The listing builds one solid part. Answer for the finished solid, in the listing's coordinates (mm). A direction names the side the tool comes from. Round coordinates to 2 decimals unless told otherwise and drop trailing zeros. Order: outer loops, then holes, each group sorted by start corner. A loop starts at its lowest first (then second) coordinate and runs counter-clockwise, first axis right, second up. Notation, with made-up numbers: (-35, -25) - (-13, -25) arc R22 ccw to (-13, 8) - close; hole circle Ø7 at (-36.75, 53). An arc over 180 degrees is marked (long way). Use CSV: the item, a comma, the result in double quotes. Start each with the question number.
Item 1: Determine the mould class of faces 1 (the cylindrical face through (847.575, 49.3, -6.509)), 2 (the flat face through (739, 49, 85)), 3 (the cylindrical face through (-39.05, 49.3, -8.67)), 4 (the cylindrical face through (882.98, 49.3, -1.87)) for opening direction X: +X half, -X half, draft (parallel to the pull), parting line (faces both ways), or undercut.
Item 2: Straight lines are drawn through the part: line 1 along X through (y, z) = (62, 0); line 2 along X through (y, z) = (68, -22); line 3 along Z through (x, y) = (282, 81.5). For each, find the intervals that lie inside material, in ascending order. Write a range as [from, to].
Item 3: Find section A-A, the plane z = 0. Give the vertices of the cut face in (x, y).
Item 4: Find section B-B, the plane y = 46. Give the vertices of the cut face in (x, z).
Item 5: Flat-ended cylindrical pins translate along their axes: P1, Ø8, axis at y = 30, z = 39, coming from the +X side; P2, Ø3, axis at x = 453.5, y = 14.5, coming from the -Z side; P3, Ø1.5, axis at y = 56.5, z = -33.5, coming from the -X side. Find the tip coordinate at first contact, or state that the pin passes through.
Item 6: Find section C-C, the plane x = 304. Give the vertices of the cut face in (y, z), plus the area to 3 significant figures.
Item 7: For faces 5 (the flat face through (403, 49, 65)), 6 (the cylindrical face through (669.13, 49.3, -70.484)), 7 (the flat face through (406, 100, 1)), determine the directions among +Z, -Z, +X, -X, +Y, -Y from which every point of the face is accessible in a straight line to the end or side of a thin tool.
```python
from build123d import *

# Parameters (mm, degrees)
SKETCH1_R           = 50
SKETCH1_R_2         = 40
BOSS_EXTRUDE1_DEPTH = 100
FILLET1_R           = 25


with BuildPart() as part:
    # Sketch1 → Boss-Extrude1 (new body)
    with BuildSketch(Plane(origin=(0, 0, 0), x_dir=(1, 0, 0), z_dir=(0, 1, 0))):
        with BuildLine():
            Line((120, 85), (120, 65))
            Line((120, 65), (678, 65))
            Line((678, 65), (678, 85))
            Line((678, 85), (798, 85))
            ThreePointArc((798, 85), (883, 0), (798, -85))
            Line((798, -85), (678, -85))
            Line((678, -85), (678, -65))
            Line((678, -65), (120, -65))
            Line((120, -65), (120, -85))
            Line((120, -85), (0, -85))
            ThreePointArc((0, -85), (-85, 0), (0, 85))
            Line((0, 85), (120, 85))
        make_face()
        with Locations(Location((798, 0, 0), (0, 0, 270))):
            Circle(SKETCH1_R, mode=Mode.SUBTRACT)
        with Locations(Location((0, 0, 0), (0, 0, 270))):
            Circle(SKETCH1_R_2, mode=Mode.SUBTRACT)
    extrude(amount=BOSS_EXTRUDE1_DEPTH)

    # Fillet1
    # the kernel refuses this fillet: 25 mm, written as the material it adds along each edge
    with BuildSketch(Plane(origin=(120, 0, 65), x_dir=(1, 0, 0), z_dir=(0, 1, 0)), Plane(origin=(678, 0, -65), x_dir=(-1, 0, 0), z_dir=(0, 1, 0))) as fillet1_piece_1:
        with BuildLine():
            CenterArc((24.494897428, -25), FILLET1_R, 90, 78.463040967)
            Line((0, -20), (-0.489897949, -19.9))
            ThreePointArc((-0.489897949, -19.9), (-0.5, -10), (-0.5, 0))
            Line((-0.5, 0), (0, 0.5))
            Line((0, 0.5), (24.494897428, 0.5))
            Line((24.494897428, 0.5), (24.494897428, 0))
        make_face()
    extrude(amount=100)
    with BuildSketch(Plane(origin=(678, 0, 65), x_dir=(0, 0, 1), z_dir=(0, 1, 0)), Plane(origin=(120, 0, -65), x_dir=(0, 0, -1), z_dir=(0, 1, 0))) as fillet1_piece_2:
        with BuildLine():
            CenterArc((25, -24.494897428), FILLET1_R, 101.536959033, 78.463040967)
            Line((0, -24.494897428), (-0.5, -24.494897428))
            Line((-0.5, -24.494897428), (-0.5, 0))
            Line((-0.5, 0), (0, 0.5))
            ThreePointArc((0, 0.5), (10, 0.5), (19.9, 0.489897949))
            Line((19.9, 0.489897949), (20, 0))
        make_face()
    extrude(amount=100)


solid = part.part
```
Worked out:
1,face 1,"undercut"
1,face 2,"draft"
1,face 3,"undercut"
1,face 4,"+X half"
2,line 1,"x = [-85, -40], [40, 748], [848, 883]"
2,line 2,"x = [-82.1, -33.41], [33.41, 753.1], [842.9, 880.1]"
2,line 3,"z = [-65, 65]"
3,outline,"(-85, 0) - (-40, 0) - (-40, 100) - (-85, 100) - close; (40, 0) - (748, 0) - (748, 100) - (40, 100) - close; (848, 0) - (883, 0) - (883, 100) - (848, 100) - close"
4,outline,"(0, -85) - (120, -85) arc R25 cw to (144.49, -65) - (653.51, -65) arc R25 cw to (678, -85) - (798, -85) arc R85 ccw to (798, 85) - (678, 85) arc R25 cw to (653.51, 65) - (144.49, 65) arc R25 cw to (120, 85) - (0, 85) arc R85 ccw to start; hole circle Ø80 at (0, 0); hole circle Ø100 at (798, 0)"
5,P1,"stops at x = 875.46"
5,P2,"stops at z = -65"
5,P3,"stops at x = -78.44"
6,outline,"(0, -65) - (100, -65) - (100, 65) - (0, 65) - close"
6,area,"13,000 mm²"
7,face 5,"+Z, +Y, -Y"
7,face 6,"-Z, +Y, -Y"
7,face 7,"+Z, -Z, +X, -X, +Y"
